```python
from build123d import *

# Parameters (mm, degrees)
EXTRUDE_1_DEPTH           = 72
CHAMFER_1_SIZE            = 3
CUT_EXTRUDE_1_DEPTH       = 75.222638056
CUT_EXTRUDE_1_DEPTH_BACK  = 0.5
SKETCH_2_W                = 17
SKETCH_2_H                = 2
HOLE_WIZARD_1_D           = 8.4
HOLE_WIZARD_1_CBORE_D     = 15
HOLE_WIZARD_1_CBORE_DEPTH = 8
CHAMFER_2_SIZE            = 0.5
CHAMFER_2_SIZE_2          = 0.558326423
CHAMFER_2_SIZE_3          = 0.456812528


with BuildPart() as part:
    # 草图1 → 凸台-拉伸1 (new body)
    with BuildSketch(Plane.XY):
        Polygon((-8.5, 0), (8.5, 0), (10, 15), (-10, 15), align=None)
    extrude(amount=-EXTRUDE_1_DEPTH)

    # 倒角1
    chamfer_1_edges = [part.edges().sort_by_distance(p)[0] for p in [
        (0, 0, 0),
    ]]
    chamfer(chamfer_1_edges, length=CHAMFER_1_SIZE)

    # 草图2 → 切除-拉伸-薄壁1 (cut, two sides: drawn at the far end of the back side and taken through both)
    with BuildSketch(Plane.XZ.offset(-CUT_EXTRUDE_1_DEPTH_BACK)):
        with Locations((0, -21)):
            Rectangle(SKETCH_2_W, SKETCH_2_H)
    extrude(amount=CUT_EXTRUDE_1_DEPTH + CUT_EXTRUDE_1_DEPTH_BACK, mode=Mode.SUBTRACT)

    # 孔1 (through all)
    with Locations(Plane(origin=(0, 15, 0), x_dir=(1, 0, 0), z_dir=(0, 1, 0))):
        with Locations((0, 34), (0, 60)):
            CounterBoreHole(HOLE_WIZARD_1_D / 2, HOLE_WIZARD_1_CBORE_D / 2, HOLE_WIZARD_1_CBORE_DEPTH)

    # 倒角2
    # the kernel refuses this chamfer: 0.558326423, 0.5, 0.456812528 mm, written as the material it takes off along each edge
    with BuildSketch(Plane(origin=(-8.5, 0, -1.560537605), x_dir=(0.9995316374096256, -0.030602382541768988, 0), z_dir=(0, 0, -1))) as chamfer_2_piece_1:
        Polygon((CHAMFER_2_SIZE * 0.99953163741, -CHAMFER_2_SIZE * 0.0306023825418), (-CHAMFER_2_SIZE_2 * 0.129907624032, -CHAMFER_2_SIZE_2 * 0.991526101843), (0, 0), align=None)
    extrude(amount=19.87892479, mode=Mode.SUBTRACT)
    with BuildSketch(Plane(origin=(8.5, 0, -1.560537605), x_dir=(-0.9996983211362673, -0.024561488499858487, 0), z_dir=(0, 0, -1))) as chamfer_2_piece_2:
        Polygon((CHAMFER_2_SIZE_2 * 0.999698321845, CHAMFER_2_SIZE_2 * 0.0245614885173), (-CHAMFER_2_SIZE * 0.123913295356, CHAMFER_2_SIZE * 0.992293049071), (0, 0), align=None)
    extrude(amount=19.87892479, mode=Mode.SUBTRACT)
    with BuildSketch(Plane(origin=(8.5, 0, -20.560537605), x_dir=(0.12990762393949729, 0.9915261011402545, 0), z_dir=(0, 0, -1))) as chamfer_2_piece_3:
        Polygon((CHAMFER_2_SIZE * 0.99953163741, -CHAMFER_2_SIZE * 0.0306023825418), (-CHAMFER_2_SIZE_2 * 0.129907624032, -CHAMFER_2_SIZE_2 * 0.991526101843), (0, 0), align=None)
    extrude(amount=52.87892479, mode=Mode.SUBTRACT)
    with BuildSketch(Plane(origin=(-8.5, 0, -20.560537605), x_dir=(-0.1239132953563816, 0.9922930490706474, 0), z_dir=(0, 0, -1))) as chamfer_2_piece_4:
        Polygon((CHAMFER_2_SIZE_2 * 0.999698321845, CHAMFER_2_SIZE_2 * 0.0245614885173), (-CHAMFER_2_SIZE * 0.123913295356, CHAMFER_2_SIZE * 0.992293049071), (0, 0), align=None)
    extrude(amount=52.87892479, mode=Mode.SUBTRACT)
    # the kernel refuses this chamfer: 0.558326423, 0.5, 0.456812528 mm, written as the material it takes off along each edge
    with BuildSketch(Plane(origin=(-10, 15, 1.285841494), x_dir=(0.07210667854261384, -0.9973969254562359, 0), z_dir=(0, 0, -1)), Plane(origin=(10, 15, 1.285841494), x_dir=(-0.9996219169112968, 0.027495876610585647, 0), z_dir=(0, 0, -1))) as chamfer_2_2_piece_1:
        Polygon((CHAMFER_2_SIZE * 0.999621916911, -CHAMFER_2_SIZE * 0.0274958766106), (CHAMFER_2_SIZE_3 * 0.0721066785794, -CHAMFER_2_SIZE_3 * 0.997396925964), (0, 0), align=None)
    extrude(amount=74.571682988, mode=Mode.SUBTRACT)


solid = part.part
```
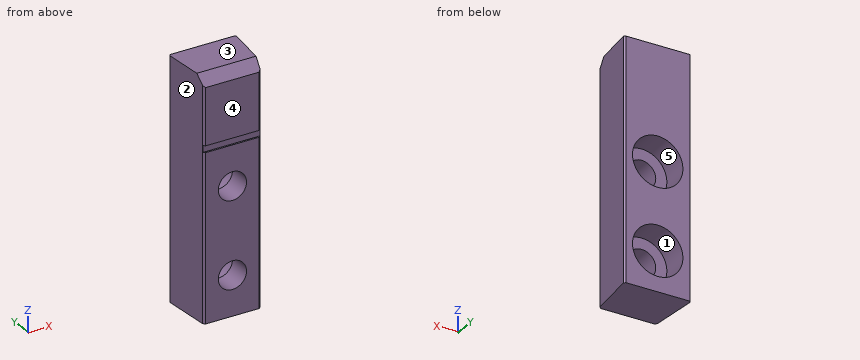
Input: part model. Units: mm. Frame: model coordinates. Face numbers are marked on the shaded views. A direction names the side the tool comes from. Coordinates: 2 decimals unless noted, no trailing zeros. Loops run counter-clockwise (first coordinate to the right, second up) from the corner with the lowest first, then second, coordinate; pieces in that order, holes last. Notation, with made-up numbers: M -24.75,1 L -8.75,1 A17 cw -8.75,5 Z; hole C -27,71.25 d11. An arc over 180 degrees is marked long. Use a Markdown table: item, result. Add a question column.
1) Pin query (flat end, axial travel): P1, Ø1, axis at x = 1, z = -21, coming from the -Y side; P2, Ø3, axis at y = 8.5, z = -37, coming from the +X side; P3, Ø1.5, axis at y = 2.5, z = -63, coming from the +X side (3 decimals). Return the tip coordinate at first contact, or that it passes through.
2) Draft query along Z for the marked faces 3, 4 and 5. Return one class per face: +Z half, -Z half, draft (parallel to the pull), parting line (faces both ways), or undercut.
3) Section B-B, the plane z = -60. Return the cut outline in (x, y).
4) Set-up query: the marked faces 1 and 2. Return all of +Z, -Z, +X, -X, +Y, -Y with unobstructed straight access to the full face (end or side cutting, diameter ignored); none if empty.
5) Section A-A, the plane x = 0. Return the cut outline in (y, z).
6) Line query: L1, parallel to Z at x = 0, y = 11.5; L2, parallel to Z at x = 0, y = 5.5; L3, parallel to Y at x = 4, z = -30. Output: solid intervals per line, ascending. Write a range as from..to.
7) Section C-C, the plane y = 2. Return the cut outline in (x, z).
8) Section D-D, the plane z = -44. Return the cut outline in (x, y).
Answer below:
| question | item | result |
|---|---|---|
| 1 | P1 | y = 0.5 |
| 1 | P2 | x = 9.5 |
| 1 | P3 | x = 8.825 |
| 2 | face 3 | +Z half |
| 2 | face 4 | draft |
| 2 | face 5 | undercut |
| 3 | outline | M -9.95,14.5 L -8.56,0.56 L -8,0 L -4.2,0 L -4.2,7 L -7.5,7 L -7.5,15 L -9.54,15 Z; M 4.2,0 L 7.94,0 L 8.55,0.5 L 9.95,14.55 L 9.5,15 L 7.5,15 L 7.5,7 L 4.2,7 Z |
| 4 | face 1 | +Y |
| 4 | face 2 | +Z, -Z, -X, -Y |
| 5 | outline | M 0,-72 L 15,-72 L 15,-67.5 L 7,-67.5 L 7,-64.2 L 0,-64.2 Z; M 0,-55.8 L 7,-55.8 L 7,-52.5 L 15,-52.5 L 15,-41.5 L 7,-41.5 L 7,-38.2 L 0,-38.2 Z; M 0,-29.8 L 7,-29.8 L 7,-26.5 L 15,-26.5 L 15,0 L 3,0 L 0,-3 L 0,-20 L 0.5,-20 L 0.5,-22 L 0,-22 Z |
| 6 | L1 | -72..-67.5, -52.5..-41.5, -26.5..0 |
| 6 | L2 | -72..-64.2, -55.8..-38.2, -29.8..0 |
| 6 | L3 | 0..7 |
| 7 | outline | M -8.7,-72 L 8.7,-72 L 8.7,-1 L -8.7,-1 Z; hole C 0,-60 d8.4; hole C 0,-34 d8.4 |
| 8 | outline | M -9.95,14.5 L -8.56,0.56 L -8,0 L 7.94,0 L 8.55,0.5 L 9.95,14.55 L 9.5,15 L -9.54,15 Z |
